Check sheet for the drawn part. Datum: minimum x, y, z corner. Units: mm. A direction names the side the tool comes from. Coordinates: 2 decimals unless noted, no trailing zeros. Order: outer loops, then holes, each group sorted by start corner. A loop starts at its lowest first (then second) coordinate and runs counter-clockwise, first axis right, second up. Notation, with made-up numbers: (3.5, 42) - (12.5, 42) arc R13 ccw to (12.5, 63) - close; hole circle Ø10 at (31.5, 14.5). An arc over 180 degrees is marked (long way). Return JSON: item names as keys, results as strings. Group by question number.
Item 1: Tool access check on the marked faces 1, 2 and 3. Record the directions out of +Z, -Z, +X, -X, +Y, -Y that give a thin tool (end or side, any length) a straight path to the whole face; none if there is none.
Item 2: Section check C-C on x = 56. Enter the section's corners in (y, z).
Item 3: Gauge pin test, flat ends, axial feed: pin 1 (4 mm diameter, centred on x = 9, y = 40.5, fed in from +Z); pin 2 (3 mm diameter, centred on y = 42, z = 65.5, fed in from +X) (1 decimal); pin 3 (2.5 mm diameter, centred on y = 38.5, z = 63.5, fed in from +X). Record the tip position at first contact, or that the pin passes through.
Item 4: Section check D-D on z = 57. Enter the section's corners in (x, y), then the cut area to 3 significant figures.
Item 5: Section check A-A on z = 25. Enter the section's corners in (x, y).
Item 6: Section check B-B on y = 46.5. Enter the section's corners in (x, z), then the cut area to 3 significant figures.
Item 7: Scan lines: probe 1 along Z at (x, y) = (88, 35.5); probe 2 along Y at (x, z) = (8.5, 50); probe 3 along Z at (x, y) = (23, 26). Record each from-to range of solid material in increasing order.
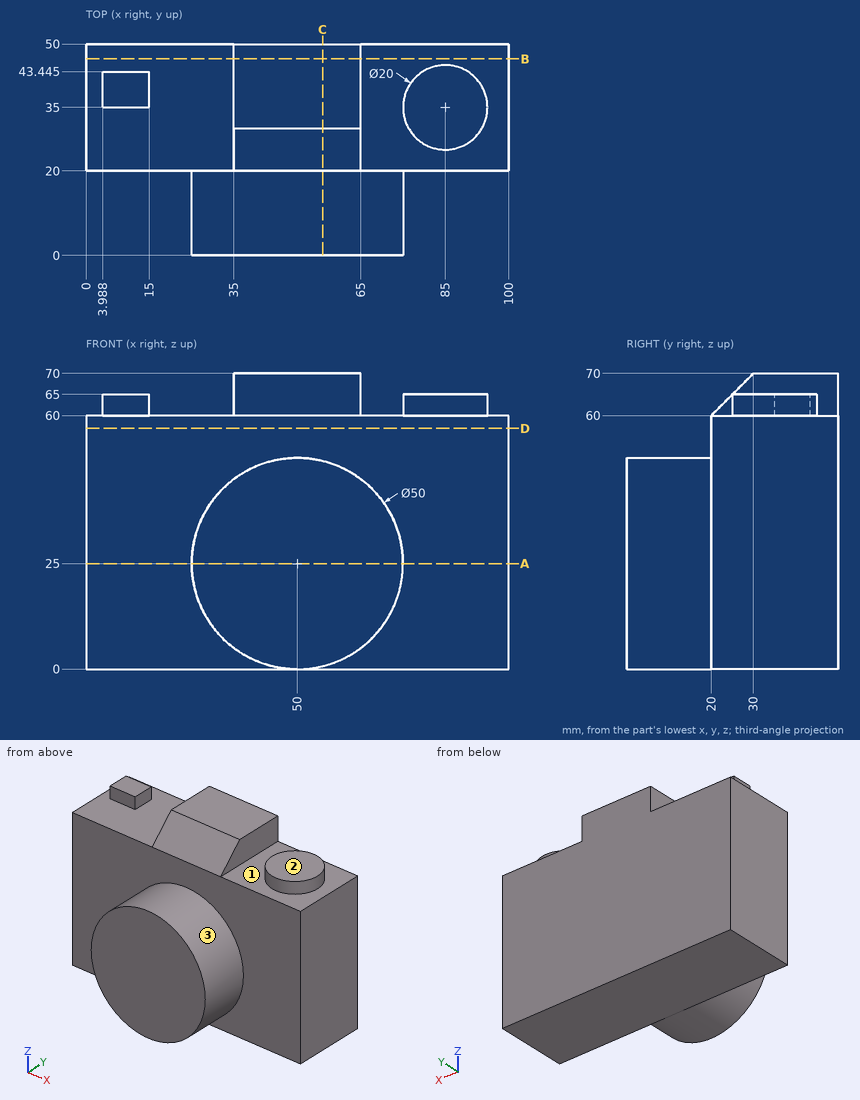
Computed:
{
 "1": {"face 1": "+Z", "face 2": "+Z, +X, +Y, -Y", "face 3": "-Y"},
 "2": {"outline": "(0, 0.73) - (20, 0.73) - (20, 0) - (50, 0) - (50, 70) - (30, 70) - (20, 60) - (20, 49.27) - (0, 49.27) - close"},
 "3": {"pin 1": "stops at z = 65", "pin 2": "stops at x = 93.3", "pin 3": "stops at x = 94.74"},
 "4": {"outline": "(0, 20) - (100, 20) - (100, 50) - (0, 50) - close", "area": "3,000 mm²"},
 "5": {"outline": "(0, 20) - (25, 20) - (25, 0) - (75, 0) - (75, 20) - (100, 20) - (100, 50) - (0, 50) - close"},
 "6": {"outline": "(0, 0) - (100, 0) - (100, 60) - (65, 60) - (65, 70) - (35, 70) - (35, 60) - (0, 60) - close", "area": "6,300 mm²"},
 "7": {"probe 1": "z = 0 to 65", "probe 2": "y = 20 to 50", "probe 3": "z = 0 to 60"}
}
